CAD build for the part. Positions are in the model's coordinates, mm. Face numbers are marked on the shaded views. A direction names the side the tool comes from. Round coordinates to 2 decimals unless told otherwise and drop trailing zeros. Order: outer loops, then holes, each group sorted by start corner. A loop starts at its lowest first (then second) coordinate and runs counter-clockwise, first axis right, second up.
```python
from build123d import *

# Parameters (mm, degrees)
ESQUISSE1_R                  = 12.5
BOSS_EXTRU_1_DEPTH           = 80
BOSS_EXTRU_2_DEPTH           = 2.5
BOSS_EXTRU_2_DEPTH_BACK      = 27.5
ESQUISSE2_W                  = 35
ESQUISSE2_H                  = 48
ENL_V_MAT_EXTRU_1_DEPTH      = 89.746830929
ENL_V_MAT_EXTRU_1_DEPTH_BACK = 89.746830929
ESQUISSE3_W                  = 35
ESQUISSE3_H                  = 18
ENL_V_MAT_EXTRU_2_DEPTH      = 95.493386012
ENL_V_MAT_EXTRU_2_DEPTH_BACK = 95.493386012
ESQUISSE4_R                  = 6


with BuildPart() as part:
    # Esquisse1 → Boss.-Extru.1 (new body)
    with BuildSketch(Plane.XY):
        Circle(ESQUISSE1_R)
    extrude(amount=BOSS_EXTRU_1_DEPTH)

    # Esquisse2 → Boss.-Extru.2 (add, two sides: drawn at the far end of the back side and taken through both)
    with BuildSketch(Plane.ZY.offset(12.5).offset(-BOSS_EXTRU_2_DEPTH_BACK)):
        with Locations((-17.5, 0)):
            Rectangle(ESQUISSE2_W, ESQUISSE2_H)
    extrude(amount=BOSS_EXTRU_2_DEPTH + BOSS_EXTRU_2_DEPTH_BACK)

    # Esquisse3 → Enl_v. mat.-Extru.1 (cut, two sides: drawn at the far end of the back side and taken through both)
    with BuildSketch(Plane.ZY.offset(15).offset(-ENL_V_MAT_EXTRU_1_DEPTH_BACK)):
        with Locations((-17.5, 0)):
            Rectangle(ESQUISSE3_W, ESQUISSE3_H)
    extrude(amount=ENL_V_MAT_EXTRU_1_DEPTH + ENL_V_MAT_EXTRU_1_DEPTH_BACK, mode=Mode.SUBTRACT)

    # Esquisse4 → Enl_v. mat.-Extru.2 (cut, two sides: drawn at the far end of the back side and taken through both)
    with BuildSketch(Plane.XZ.offset(24).offset(-ENL_V_MAT_EXTRU_2_DEPTH_BACK)):
        with Locations(Location((0, -17.5, 0), (0, 0, 270))):
            Circle(ESQUISSE4_R)
    extrude(amount=ENL_V_MAT_EXTRU_2_DEPTH + ENL_V_MAT_EXTRU_2_DEPTH_BACK, mode=Mode.SUBTRACT)


solid = part.part
```
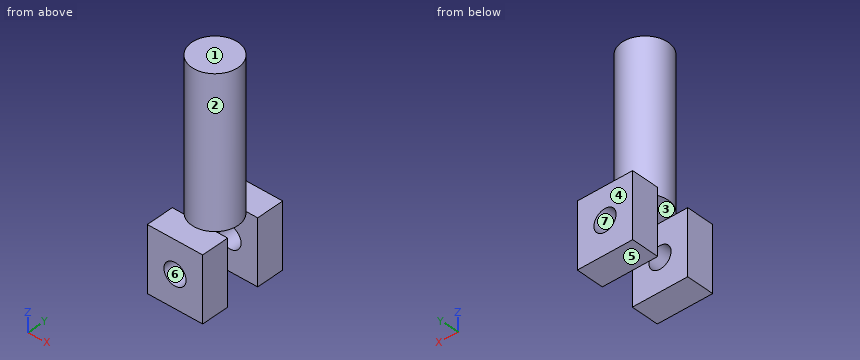
1. Cut at B-B, the plane x = 0. Write the cut outline in (y, z), and give its area (3 significant figures).
2. Cut at C-C, the plane z = 12.5. Write the cut outline in (x, y), and give its area (3 significant figures).
3. Tool access for the marked faces 1, 2 and 3: list every direction of +Z, -Z, +X, -X, +Y, -Y with a clear straight run to the whole face (end or side of a thin tool).
4. Cut at D-D, the plane y = -3.5. Write the cut outline in (x, z).
5. Pin check, flat tips, straight feed: P1, Ø4, axis at x = -8, z = 65, coming from the +Y side; P2, Ø10, axis at y = -19, z = 23.5, coming from the +X side; P3, Ø10, axis at x = -11.5, z = 20, coming from the -Y side; P4, Ø12, axis at y = -9.5, z = 45, coming from the -X side. Stop position of each tip, or through.
6. Cut at A-A, the plane z = -17.5. Write the cut outline in (x, y).
7. Drill centre lines: line 1 (X direction, y = -17, z = -17); line 2 (Y direction, x = -1.75, z = -3); line 3 (Z direction, x = 0, y = -15). Where is each one in solid material? Low to high.
8. Mould opens along Z. For the marked faces 4, 5, 6 and 7 say: released by +Z, released by -Z, zero draft, split by the parting line, or undercut.
Outcome:
1. outline: (-24, -35) - (-9, -35) - (-9, -23.5) - (-24, -23.5) - close; (-24, -11.5) - (-9, -11.5) - (-9, 0) - (9, 0) - (9, -11.5) - (24, -11.5) - (24, 0) - (12.5, 0) - (12.5, 80) - (-12.5, 80) - (-12.5, 0) - (-24, 0) - close; (9, -35) - (24, -35) - (24, -23.5) - (9, -23.5) - close
1. area: 2,690 mm2
2. outline: circle Ø25 at (0, 0)
2. area: 491 mm2
3. face 1: +Z, +X, -X, +Y, -Y
3. face 2: +Z
3. face 3: -Z, +X, -X
4. outline: (-12, 0) - (12, 0) - (12, 80) - (-12, 80) - close
5. P1: stops at y = 10.97
5. P2: passes through
5. P3: stops at y = -10.68
5. P4: stops at x = -12
6. outline: (-15, -24) - (-6, -24) - (-6, -9) - (-15, -9) - close; (-15, 9) - (-6, 9) - (-6, 24) - (-15, 24) - close; (6, -24) - (15, -24) - (15, -9) - (6, -9) - close; (6, 9) - (15, 9) - (15, 24) - (6, 24) - close
7. line 1: x = -15 to -5.98, 5.98 to 15
7. line 2: y = -24 to -9, 9 to 24
7. line 3: z = -35 to -23.5, -11.5 to 0
8. face 4: zero draft
8. face 5: released by -Z
8. face 6: undercut
8. face 7: undercut
